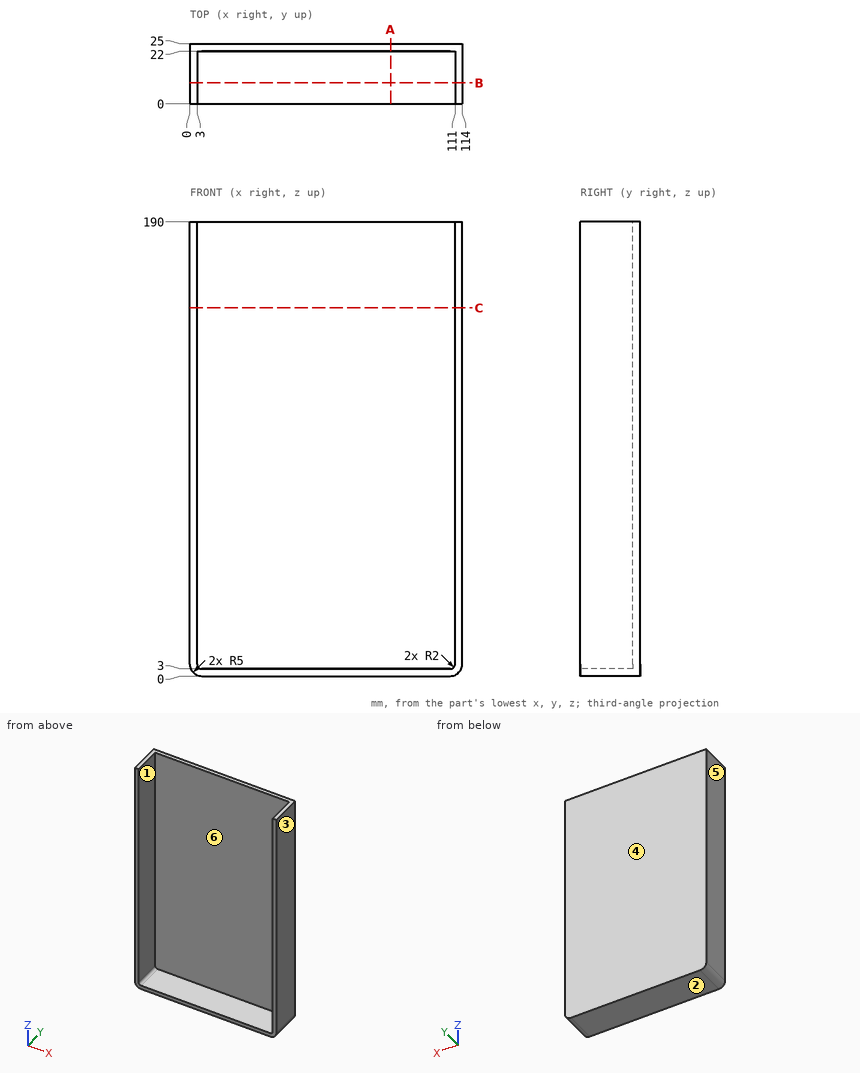
Geometry check sheet. Reference: drawing and pictorial views, mm from the part's lowest x, y, z. A direction names the side the tool comes from. Round coordinates to 2 decimals unless told otherwise and drop trailing zeros. Order: outer loops, then holes, each group sorted by start corner. A loop starts at its lowest first (then second) coordinate and runs counter-clockwise, first axis right, second up. Notation, with made-up numbers: (-21, 51) - (-12, 51) arc R14 cw to (-12, 75) - close; hole circle Ø1 at (-5, 78.25). An arc over 180 degrees is marked (long way). One line per question, with ' | ' between items. Start each with the question number.
(1) Sectioned sample at B-B on y = 8.75. Record the cut outline in (x, z).
(2) Sectioned sample at C-C on z = 154. Record the cut outline in (x, y), and give its area (3 significant figures).
(3) Thickness scan on L1, parallel to X at y = 20.5, z = 146; L2, parallel to Z at x = 21, y = 2; L3, parallel to Y at x = 28.5, z = 65. Record the ranges inside material, lowest first. Write a range as [from, to].
(4) Sectioned sample at A-A on x = 84. Record the cut outline in (y, z), and give its area (3 significant figures).
(5) Release check for a two-part mould opening along X. For the marked faces 3, 4, 5 and 6 record: released by +X, released by -X, zero draft, split by the parting line, or undercut.
(6) Access from +Z, -Z, +X, -X, +Y, -Y to the whole of each face (thin tool, end or side, straight path). Record for the marked faces 1 and 2.
(7) Depth check by flat-ended pin: pin 1 Ø5 at (x, z) = (91.5, 118) entering from -Y; pin 2 Ø10 at (y, z) = (18.5, 21.5) entering from -X. Enter the tip coordinate at first touch or a pass-through.
Conclusion:
1) outline: (0, 5) arc R5 ccw to (5, 0) - (109, 0) arc R5 ccw to (114, 5) - (114, 190) - (111, 190) - (111, 5) arc R2 cw to (109, 3) - (5, 3) arc R2 cw to (3, 5) - (3, 190) - (0, 190) - close
2) outline: (0, 0) - (3, 0) - (3, 22) - (111, 22) - (111, 0) - (114, 0) - (114, 25) - (0, 25) - close | area: 474 mm2
3) L1: x = [0, 3], [111, 114] | L2: z = [0, 3] | L3: y = [22, 25]
4) outline: (0, 0) - (25, 0) - (25, 190) - (22, 190) - (22, 3) - (0, 3) - close | area: 636 mm2
5) face 3: released by +X | face 4: zero draft | face 5: released by -X | face 6: undercut
6) face 1: +Z, -Y | face 2: -Z, +X, -X, +Y, -Y
7) pin 1: stops at y = 22 | pin 2: stops at x = 0
